Source: CAD feature listing. Evaluate the final solid. Frame: model axes, mm. Face numbers are marked on the shaded views. A direction names the side the tool comes from. Give positions to 0.01 mm unless a question says otherwise; leave off trailing zeros. Order: outer loops, then holes, each group sorted by start corner. A loop starts at its lowest first (then second) coordinate and runs counter-clockwise, first axis right, second up. Notation, with made-up numbers: (42, 26) -> (52, 26) arc R15 ccw to (52, 43) -> close; hole circle Ø6 at (40, -17). An arc over 180 degrees is marked (long way). Use CSV: the item, a comma, the result in double quotes.
```python
from build123d import *

# Parameters (mm, degrees)
SKETCH_1_W               = 30
SKETCH_1_H               = 22.307
EXTRUDE_1_DEPTH          = 2.5
EXTRUDE_START            = -5
SKETCH_4_W               = 30
SKETCH_4_H               = 3.8465
EXTRUDE_5_DEPTH          = 30
SKETCH_5_R               = 2.5
CUT_EXTRUDE_1_DEPTH      = 44.373378932
SKETCH_6_W               = 30
SKETCH_6_H               = 25.44
EXTRUDE_6_DEPTH          = 300
SKETCH_8_W               = 30
SKETCH_8_H               = 30
EXTRUDE_8_DEPTH          = 30
SKETCH_10_W              = 100
SKETCH_10_H              = 300
EXTRUDE_9_DEPTH          = 60
FILLET_1_R               = 200
FILLET_2_R               = 200
CUT_EXTRUDE_3_DEPTH      = 461.388584133
CUT_EXTRUDE_3_DEPTH_BACK = 461.388584133


with BuildPart() as part:
    # 草图1 → 凸台-拉伸1 (new, symmetric)
    with BuildSketch(Plane(origin=(0, 0, 0), x_dir=(1, 0, 0), z_dir=(0, 1, 0))):
        Rectangle(SKETCH_1_W, SKETCH_1_H)
    extrude(amount=EXTRUDE_1_DEPTH, both=True)

    # 草图4 → 凸台-拉伸5 (add)
    with BuildSketch(Plane(origin=(0, 2.5, 0), x_dir=(1, 0, 0), z_dir=(0, 1, 0)).offset(EXTRUDE_START)):
        with Locations((0, -13.07675)):
            Rectangle(SKETCH_4_W, SKETCH_4_H)
        with Locations((0, 13.07675)):
            Rectangle(SKETCH_4_W, SKETCH_4_H)
    extrude(amount=EXTRUDE_5_DEPTH)

    # 草图5 → 切除-拉伸1 (cut, through all)
    with BuildSketch(Plane.XY.offset(15)):
        with Locations((0, 13.784)):
            Circle(SKETCH_5_R)
    extrude(amount=-CUT_EXTRUDE_1_DEPTH, mode=Mode.SUBTRACT)

    # 草图6 → 凸台-拉伸6 (add)
    with BuildSketch(Plane.XZ.offset(2.5)):
        Rectangle(SKETCH_6_W, SKETCH_6_H)
    extrude(amount=EXTRUDE_6_DEPTH)

    # 草图8 → 凸台-拉伸8 (add)
    with BuildSketch(Plane(origin=(0, 0, -12.72), x_dir=(-1, 0, 0), z_dir=(0, 0, -1))):
        with Locations((0, -287.5)):
            Rectangle(SKETCH_8_W, SKETCH_8_H)
    extrude(amount=EXTRUDE_8_DEPTH)

    # 草图10 → 凸台-拉伸9 (add)
    with BuildSketch(Plane(origin=(0, 0, -42.72), x_dir=(-1, 0, 0), z_dir=(0, 0, -1))):
        with Locations((0, -287.5)):
            Rectangle(SKETCH_10_W, SKETCH_10_H)
    extrude(amount=EXTRUDE_9_DEPTH)

    # 圆角1
    # the kernel refuses this fillet: 200 mm, written as the material it takes off along each edge
    with BuildSketch(Plane(origin=(-407.071421427, -437.5, -42.72), x_dir=(0, 1, 0), z_dir=(1, 0, 0))) as fillet_1_piece_1_section:
        with BuildLine():
            CenterArc((142.828568571, -200), FILLET_1_R, 90, 45.572995999)
            Line((0, -60), (-2.856571371, -57.2))
            ThreePointArc((-2.856571371, -57.2), (-4, -30), (-4, 0))
            Line((-4, 0), (0, 4))
            Line((0, 4), (142.828568571, 4))
            Line((142.828568571, 4), (142.828568571, 0))
        make_face()
    fillet_1_piece_1 = extrude(amount=814.142842854, mode=Mode.PRIVATE)
    fillet_1_piece_1 = split(fillet_1_piece_1, bisect_by=Plane(origin=(-211.035710714, -302.5, -40.745799624), z_dir=(0, 1, 0)), keep=Keep.TOP, mode=Mode.PRIVATE)
    fillet_1_piece_1 = split(fillet_1_piece_1, bisect_by=Plane(origin=(-15, -298.610396999, -40.745799624), z_dir=(-1, 0, 0)), keep=Keep.TOP, mode=Mode.PRIVATE)
    add(fillet_1_piece_1, mode=Mode.SUBTRACT)
    with BuildSketch(Plane(origin=(-407.071421427, -437.5, -42.72), x_dir=(0, 1, 0), z_dir=(1, 0, 0))) as fillet_1_piece_2_section:
        with BuildLine():
            CenterArc((142.828568571, -200), FILLET_1_R, 90, 45.572995999)
            Line((0, -60), (-2.856571371, -57.2))
            ThreePointArc((-2.856571371, -57.2), (-4, -30), (-4, 0))
            Line((-4, 0), (0, 4))
            Line((0, 4), (142.828568571, 4))
            Line((142.828568571, 4), (142.828568571, 0))
        make_face()
    fillet_1_piece_2 = extrude(amount=814.142842854, mode=Mode.PRIVATE)
    fillet_1_piece_2 = split(fillet_1_piece_2, bisect_by=Plane(origin=(-211.035710714, -302.5, -57.711003377), z_dir=(0, -1, 0)), keep=Keep.TOP, mode=Mode.PRIVATE)
    fillet_1_piece_2 = split(fillet_1_piece_2, bisect_by=Plane(origin=(-15, -400.231636696, -57.711003377), z_dir=(-1, 0, 0)), keep=Keep.TOP, mode=Mode.PRIVATE)
    add(fillet_1_piece_2, mode=Mode.SUBTRACT)
    with BuildSketch(Plane(origin=(-407.071421427, -437.5, -42.72), x_dir=(0, 1, 0), z_dir=(1, 0, 0))) as fillet_1_piece_3_section:
        with BuildLine():
            CenterArc((142.828568571, -200), FILLET_1_R, 90, 45.572995999)
            Line((0, -60), (-2.856571371, -57.2))
            ThreePointArc((-2.856571371, -57.2), (-4, -30), (-4, 0))
            Line((-4, 0), (0, 4))
            Line((0, 4), (142.828568571, 4))
            Line((142.828568571, 4), (142.828568571, 0))
        make_face()
    fillet_1_piece_3 = extrude(amount=814.142842854, mode=Mode.PRIVATE)
    fillet_1_piece_3 = split(fillet_1_piece_3, bisect_by=Plane(origin=(0, -302.5, -57.711003377), z_dir=(0, -1, 0)), keep=Keep.TOP, mode=Mode.PRIVATE)
    fillet_1_piece_3 = split(fillet_1_piece_3, bisect_by=Plane(origin=(15, -400.231636696, -57.711003377), z_dir=(-1, 0, 0)), keep=Keep.TOP, mode=Mode.PRIVATE)
    fillet_1_piece_3 = split(fillet_1_piece_3, bisect_by=Plane(origin=(-15, -400.231636696, -57.711003377), z_dir=(1, 0, 0)), keep=Keep.TOP, mode=Mode.PRIVATE)
    add(fillet_1_piece_3, mode=Mode.SUBTRACT)
    with BuildSketch(Plane(origin=(-407.071421427, -437.5, -42.72), x_dir=(0, 1, 0), z_dir=(1, 0, 0))) as fillet_1_piece_4_section:
        with BuildLine():
            CenterArc((142.828568571, -200), FILLET_1_R, 90, 45.572995999)
            Line((0, -60), (-2.856571371, -57.2))
            ThreePointArc((-2.856571371, -57.2), (-4, -30), (-4, 0))
            Line((-4, 0), (0, 4))
            Line((0, 4), (142.828568571, 4))
            Line((142.828568571, 4), (142.828568571, 0))
        make_face()
    fillet_1_piece_4 = extrude(amount=814.142842854, mode=Mode.PRIVATE)
    fillet_1_piece_4 = split(fillet_1_piece_4, bisect_by=Plane(origin=(211.035710714, -302.5, -40.745799624), z_dir=(0, 1, 0)), keep=Keep.TOP, mode=Mode.PRIVATE)
    fillet_1_piece_4 = split(fillet_1_piece_4, bisect_by=Plane(origin=(15, -298.610396999, -40.745799624), z_dir=(1, 0, 0)), keep=Keep.TOP, mode=Mode.PRIVATE)
    add(fillet_1_piece_4, mode=Mode.SUBTRACT)
    with BuildSketch(Plane(origin=(-407.071421427, -437.5, -42.72), x_dir=(0, 1, 0), z_dir=(1, 0, 0))) as fillet_1_piece_5_section:
        with BuildLine():
            CenterArc((142.828568571, -200), FILLET_1_R, 90, 45.572995999)
            Line((0, -60), (-2.856571371, -57.2))
            ThreePointArc((-2.856571371, -57.2), (-4, -30), (-4, 0))
            Line((-4, 0), (0, 4))
            Line((0, 4), (142.828568571, 4))
            Line((142.828568571, 4), (142.828568571, 0))
        make_face()
    fillet_1_piece_5 = extrude(amount=814.142842854, mode=Mode.PRIVATE)
    fillet_1_piece_5 = split(fillet_1_piece_5, bisect_by=Plane(origin=(211.035710714, -302.5, -57.711003377), z_dir=(0, -1, 0)), keep=Keep.TOP, mode=Mode.PRIVATE)
    fillet_1_piece_5 = split(fillet_1_piece_5, bisect_by=Plane(origin=(15, -400.231636696, -57.711003377), z_dir=(1, 0, 0)), keep=Keep.TOP, mode=Mode.PRIVATE)
    add(fillet_1_piece_5, mode=Mode.SUBTRACT)

    # 圆角2
    # the kernel refuses this fillet: 200 mm, written as the material it takes off along each edge
    with BuildSketch(Plane(origin=(407.071421427, -137.5, -42.72), x_dir=(0, 0, -1), z_dir=(-1, 0, 0))) as fillet_2_piece_1_section:
        with BuildLine():
            CenterArc((200, 142.828568571), FILLET_2_R, 180, 45.572995999)
            Line((0, 142.828568571), (-4, 142.828568571))
            Line((-4, 142.828568571), (-4, 0))
            Line((-4, 0), (0, -4))
            ThreePointArc((0, -4), (30, -4), (57.2, -2.856571371))
            Line((57.2, -2.856571371), (60, 0))
        make_face()
    fillet_2_piece_1 = extrude(amount=814.142842854, mode=Mode.PRIVATE)
    fillet_2_piece_1 = split(fillet_2_piece_1, bisect_by=Plane(origin=(15, -174.768363304, -57.711003377), z_dir=(1, 0, 0)), keep=Keep.TOP, mode=Mode.PRIVATE)
    fillet_2_piece_1 = split(fillet_2_piece_1, bisect_by=Plane(origin=(211.035710714, -272.5, -57.711003377), z_dir=(0, 1, 0)), keep=Keep.TOP, mode=Mode.PRIVATE)
    add(fillet_2_piece_1, mode=Mode.SUBTRACT)
    with BuildSketch(Plane(origin=(407.071421427, -137.5, -42.72), x_dir=(0, 0, -1), z_dir=(-1, 0, 0))) as fillet_2_piece_2_section:
        with BuildLine():
            CenterArc((200, 142.828568571), FILLET_2_R, 180, 45.572995999)
            Line((0, 142.828568571), (-4, 142.828568571))
            Line((-4, 142.828568571), (-4, 0))
            Line((-4, 0), (0, -4))
            ThreePointArc((0, -4), (30, -4), (57.2, -2.856571371))
            Line((57.2, -2.856571371), (60, 0))
        make_face()
    fillet_2_piece_2 = extrude(amount=814.142842854, mode=Mode.PRIVATE)
    fillet_2_piece_2 = split(fillet_2_piece_2, bisect_by=Plane(origin=(15, -276.389603001, -40.745799624), z_dir=(1, 0, 0)), keep=Keep.TOP, mode=Mode.PRIVATE)
    fillet_2_piece_2 = split(fillet_2_piece_2, bisect_by=Plane(origin=(211.035710714, -272.5, -40.745799624), z_dir=(0, -1, 0)), keep=Keep.TOP, mode=Mode.PRIVATE)
    add(fillet_2_piece_2, mode=Mode.SUBTRACT)
    with BuildSketch(Plane(origin=(407.071421427, -137.5, -42.72), x_dir=(0, 0, -1), z_dir=(-1, 0, 0))) as fillet_2_piece_3_section:
        with BuildLine():
            CenterArc((200, 142.828568571), FILLET_2_R, 180, 45.572995999)
            Line((0, 142.828568571), (-4, 142.828568571))
            Line((-4, 142.828568571), (-4, 0))
            Line((-4, 0), (0, -4))
            ThreePointArc((0, -4), (30, -4), (57.2, -2.856571371))
            Line((57.2, -2.856571371), (60, 0))
        make_face()
    fillet_2_piece_3 = extrude(amount=814.142842854, mode=Mode.PRIVATE)
    fillet_2_piece_3 = split(fillet_2_piece_3, bisect_by=Plane(origin=(15, -174.768363304, -57.711003377), z_dir=(-1, 0, 0)), keep=Keep.TOP, mode=Mode.PRIVATE)
    fillet_2_piece_3 = split(fillet_2_piece_3, bisect_by=Plane(origin=(0, -272.5, -57.711003377), z_dir=(0, 1, 0)), keep=Keep.TOP, mode=Mode.PRIVATE)
    fillet_2_piece_3 = split(fillet_2_piece_3, bisect_by=Plane(origin=(-15, -174.768363304, -57.711003377), z_dir=(1, 0, 0)), keep=Keep.TOP, mode=Mode.PRIVATE)
    add(fillet_2_piece_3, mode=Mode.SUBTRACT)
    with BuildSketch(Plane(origin=(407.071421427, -137.5, -42.72), x_dir=(0, 0, -1), z_dir=(-1, 0, 0))) as fillet_2_piece_4_section:
        with BuildLine():
            CenterArc((200, 142.828568571), FILLET_2_R, 180, 45.572995999)
            Line((0, 142.828568571), (-4, 142.828568571))
            Line((-4, 142.828568571), (-4, 0))
            Line((-4, 0), (0, -4))
            ThreePointArc((0, -4), (30, -4), (57.2, -2.856571371))
            Line((57.2, -2.856571371), (60, 0))
        make_face()
    fillet_2_piece_4 = extrude(amount=814.142842854, mode=Mode.PRIVATE)
    fillet_2_piece_4 = split(fillet_2_piece_4, bisect_by=Plane(origin=(-211.035710714, -272.5, -57.711003377), z_dir=(0, 1, 0)), keep=Keep.TOP, mode=Mode.PRIVATE)
    fillet_2_piece_4 = split(fillet_2_piece_4, bisect_by=Plane(origin=(-15, -174.768363304, -57.711003377), z_dir=(-1, 0, 0)), keep=Keep.TOP, mode=Mode.PRIVATE)
    add(fillet_2_piece_4, mode=Mode.SUBTRACT)
    with BuildSketch(Plane(origin=(407.071421427, -137.5, -42.72), x_dir=(0, 0, -1), z_dir=(-1, 0, 0))) as fillet_2_piece_5_section:
        with BuildLine():
            CenterArc((200, 142.828568571), FILLET_2_R, 180, 45.572995999)
            Line((0, 142.828568571), (-4, 142.828568571))
            Line((-4, 142.828568571), (-4, 0))
            Line((-4, 0), (0, -4))
            ThreePointArc((0, -4), (30, -4), (57.2, -2.856571371))
            Line((57.2, -2.856571371), (60, 0))
        make_face()
    fillet_2_piece_5 = extrude(amount=814.142842854, mode=Mode.PRIVATE)
    fillet_2_piece_5 = split(fillet_2_piece_5, bisect_by=Plane(origin=(-211.035710714, -272.5, -40.745799624), z_dir=(0, -1, 0)), keep=Keep.TOP, mode=Mode.PRIVATE)
    fillet_2_piece_5 = split(fillet_2_piece_5, bisect_by=Plane(origin=(-15, -276.389603001, -40.745799624), z_dir=(-1, 0, 0)), keep=Keep.TOP, mode=Mode.PRIVATE)
    add(fillet_2_piece_5, mode=Mode.SUBTRACT)

    # 草图11 → 切除-拉伸3 (cut, two sides: drawn at the far end of the back side and taken through both)
    with BuildSketch(Plane(origin=(50, 0, 0), x_dir=(0, 0, -1), z_dir=(1, 0, 0)).offset(-CUT_EXTRUDE_3_DEPTH_BACK)):
        with BuildLine():
            Line((590.156631814, 440.987720299), (102.72, -215.998843293))
            ThreePointArc((102.72, -215.998843293), (79.092115208, -287.5), (102.72, -359.001156707))
            Line((102.72, -359.001156707), (590.156631814, -1015.987720299))
            Line((590.156631814, -1015.987720299), (2226.281095019, -1015.987720299))
            Line((2226.281095019, -1015.987720299), (2226.281095019, 440.987720299))
            Line((2226.281095019, 440.987720299), (590.156631814, 440.987720299))
        make_face()
    extrude(amount=CUT_EXTRUDE_3_DEPTH + CUT_EXTRUDE_3_DEPTH_BACK, mode=Mode.SUBTRACT)


solid = part.part
```
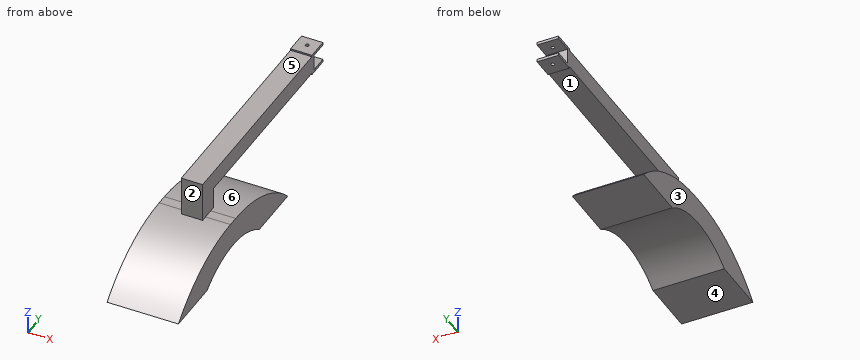
1. Access query for the marked faces 1, 2 and 3. Directions: +Z, -Z, +X, -X, +Y, -Y. A direction counts if a zero-diameter tool reaches every point of the face in a straight line with its end or side. Return the directions, or none.
Answer below:
face 1,"+X, -X"
face 2,"+Z, +X, -X, -Y"
face 3,"+Z, -Z, -X, +Y, -Y"
2. Ray query, line 1 along Y through (x, z) = (0, -12.8); line 2 along Y through (x, z) = (0, 12.35); line 3 along Y through (x, z) = (0, 13). Return the intervals inside material, ascending.
Answer below:
line 1,"y = -302.5 to -272.5, -2.5 to 11.28, 16.28 to 27.5"
line 2,"y = -302.5 to 11.28, 16.28 to 27.5"
line 3,"y = -2.5 to 11.28, 16.28 to 27.5"
3. Section query B-B on y = -178. Return loops of the section in (x, z).
Answer below:
outline,"(-50, -102.72) -> (50, -102.72) -> (50, -70.88) -> (-50, -70.88) -> close; (-15, -12.72) -> (15, -12.72) -> (15, 12.72) -> (-15, 12.72) -> close"
4. Section query D-D on x = -32.5. Return loops of the section in (y, z), plus the area to 3 significant figures.
Answer below:
outline,"(-437.5, -102.72) -> (-359, -102.72) arc R120 cw to (-216, -102.72) -> (-137.5, -102.72) arc R200 ccw to (-280.33, -42.72) -> (-294.67, -42.72) arc R200 ccw to start"
area,"10,400 mm²"
5. Section query C-C on z = -4. Return loops of the section in (x, y).
Answer below:
outline,"(-15, -302.5) -> (15, -302.5) -> (15, 2.5) -> (-15, 2.5) -> close"
6. Section query A-A on x = 7. Return loops of the section in (y, z), plus the area to 3 significant figures.
Answer below:
outline,"(-437.5, -102.72) -> (-359, -102.72) arc R120 cw to (-216, -102.72) -> (-137.5, -102.72) arc R200 ccw to (-272.5, -42.87) -> (-272.5, -12.72) -> (-2.5, -12.72) -> (-2.5, -15) -> (27.5, -15) -> (27.5, -11.15) -> (2.5, -11.15) -> (2.5, 11.15) -> (27.5, 11.15) -> (27.5, 15) -> (-2.5, 15) -> (-2.5, 12.72) -> (-302.5, 12.72) -> (-302.5, -42.87) arc R200 ccw to start"
area,"19,300 mm²"
7. Pin query (flat end, axial travel): P1, Ø2.5, axis at x = -5, z = 13.5, coming from the -Y side; P2, Ø17.5, axis at y = -143.5, z = -7, coming from the +X side; P3, Ø5, axis at x = -18, y = -369.5, coming from the +Z side. Return the tip coordinate at first contact, or that it passes through.
Answer below:
P1,"stops at y = -302.5"
P2,"stops at x = 15"
P3,"stops at z = -56.26"
8. Mould query, pull axis Z, two halves, no side actions, for the marked faces 4, 5 and 6. Classes: released by +Z, released by -Z, zero draft, split by the parting line, or undercut.
Answer below:
face 4,"released by -Z"
face 5,"released by +Z"
face 6,"undercut"
